from build123d import *

# Parameters (mm, degrees)
F0_W     = 93.846314
F0_H     = 44.516842
F0_W_2   = 89.889378
F0_H_2   = 40.80934
F1_DEPTH = 5
F2_W     = 12.35856
F2_H     = 6.520443
F2_W_2   = 6.827742
F2_H_2   = 7.738157
F2_W_3   = 6.702413
F2_H_3   = 7.531111
F3_DEPTH = 1


with BuildPart() as f1:
    # F0 (on Top) → F1 (new body)
    with BuildSketch(Plane.XY):
        Rectangle(F0_W, F0_H)
        Rectangle(F0_W_2, F0_H_2, mode=Mode.SUBTRACT)
    extrude(amount=F1_DEPTH)

    # F2 (on Top) → F3 (join)
    with BuildSketch(Plane.XY):
        with Locations((0, 18.721528)):
            Rectangle(F2_W, F2_H)
        with Locations((-26.51052, -17.850101)):
            Rectangle(F2_W_2, F2_H_2)
        with Locations((27.371847, -17.746578)):
            Rectangle(F2_W_3, F2_H_3)
    extrude(amount=F3_DEPTH)


solid = f1.part
Design review of the part built by this model. Coordinates are the model's own, in mm. A direction names the side the tool comes from. Round coordinates to 2 decimals unless told otherwise and drop trailing zeros. Loops run counter-clockwise (first coordinate to the right, second up) from the corner with the lowest first, then second, coordinate; pieces in that order, holes last. Notation, with made-up numbers: (21, 8) - (50, 8) arc R27 cw to (50, 38) - close; hole circle Ø9 at (12, 86). An arc over 180 degrees is marked (long way). One line per item, written item: value. Start each with the question number.
1) Draft analysis for pull direction X (two halves, no side actions). For faces 1 (the flat face through (46.923, 0, 2)), 2 (the flat face through (-1, -20.405, 2)), 3 (the flat face through (0, 17, 0)), state which applies: +X half, -X half, draft (parallel to the pull), parting line (faces both ways), or undercut.
2) Consider section C-C on z = 2.9. Give the boundary of the cut face in (x, y), then the cut area to 3 significant figures.
3) For faces 4 (the flat face through (-1, 22.258, 2)), 5 (the flat face through (-44.945, 0, 2)), 6 (the flat face through (-27, -17, 1)), list the 3-axis set-ups (+Z, -Z, +X, -X, +Y, -Y) from which the entire face can be reached by the end or side of a thin tool; tool diameter is ignored.
4) Consider section B-B on y = 4. Give the boundary of the cut face in (x, z), then the cut area to 3 significant figures.
5) To check wall thickness, follow L1, parallel to Y at x = 13, z = 2.3; L2, parallel to X at y = -13, z = 1.2. State the ranges of each line that lie inside material, in increasing order. Write a range as from..to.
6) Consider section A-A on x = 2.5. Give the boundary of the cut face in (y, z).
7) Consider section D-D on y = 18.5. Give the boundary of the cut face in (x, z).
8) Insertion check: pin 1 Ø3 at (x, y) = (28, -18) entering from +Z; pin 2 Ø1.5 at (x, y) = (7.5, 15.5) entering from -Z. Each pin has a flat end and moves straight along its axis. Give the tip position at first contact, or say it passes through.
Reported:
1. face 1: +X half
1. face 2: undercut
1. face 3: draft
2. outline: (-46.92, -22.26) - (46.92, -22.26) - (46.92, 22.26) - (-46.92, 22.26) - close; hole (-44.94, -20.4) - (44.94, -20.4) - (44.94, 20.4) - (-44.94, 20.4) - close
2. area: 509 mm^2
3. face 4: +Z, -Z, +X, -X, +Y
3. face 5: +Z, -Z
3. face 6: +Z
4. outline: (-46.92, 0) - (-44.94, 0) - (-44.94, 5) - (-46.92, 5) - close; (44.94, 0) - (46.92, 0) - (46.92, 5) - (44.94, 5) - close
4. area: 19.8 mm^2
5. L1: y = -22.26..-20.4, 20.4..22.26
5. L2: x = -46.92..-44.94, 44.94..46.92
6. outline: (-22.26, 0) - (-20.4, 0) - (-20.4, 5) - (-22.26, 5) - close; (15.46, 0) - (22.26, 0) - (22.26, 5) - (20.4, 5) - (20.4, 1) - (15.46, 1) - close
7. outline: (-46.92, 0) - (-44.94, 0) - (-44.94, 5) - (-46.92, 5) - close; (-6.18, 0) - (6.18, 0) - (6.18, 1) - (-6.18, 1) - close; (44.94, 0) - (46.92, 0) - (46.92, 5) - (44.94, 5) - close
8. pin 1: stops at z = 1
8. pin 2: passes through
